The listing builds one solid part. Answer for the finished solid, in the listing's coordinates (mm). A direction names the side the tool comes from. Give positions to 0.01 mm unless a question says otherwise; leave off trailing zeros. Order: outer loops, then holes, each group sorted by start corner. A loop starts at its lowest first (then second) coordinate and runs counter-clockwise, first axis right, second up. Notation, with made-up numbers: (-29.5, 53) - (-7.5, 53) arc R7 ccw to (-7.5, 64) - close; hole circle Ø3 at (82.25, 80.5). An arc over 180 degrees is marked (long way). Use CSV: the item, a comma, the result in double quotes.
```python
from build123d import *

# Parameters (mm, degrees)
CROQUIS1_R                = 4
CROQUIS1_R_2              = 2
SALIENTE_EXTRUIR1_DEPTH   = 4
SALIENTE_EXTRUIR1_2_DEPTH = 4
SALIENTE_EXTRUIR1_3_DEPTH = 4
SALIENTE_EXTRUIR1_4_DEPTH = 4
SALIENTE_EXTRUIR1_5_DEPTH = 4
CROQUIS3_R                = 2
SALIENTE_EXTRUIR4_DEPTH   = 3
CROQUIS4_R                = 4
CROQUIS4_R_2              = 2
CORTAR_EXTRUIR1_DEPTH     = 4
CROQUIS5_R                = 2
SALIENTE_EXTRUIR5_DEPTH   = 3
CROQUIS6_R                = 4
CROQUIS6_R_2              = 2
SALIENTE_EXTRUIR6_DEPTH   = 3


with BuildPart() as part:
    # Croquis1 → Saliente-Extruir1 (new body)
    with BuildSketch(Plane(origin=(0, 0, 0), x_dir=(1, 0, 0), z_dir=(0, 1, 0))):
        with Locations(Location((0, 0, 0), (0, 0, 270))):
            Circle(CROQUIS1_R)
        with Locations(Location((0, 0, 0), (0, 0, 270))):
            Circle(CROQUIS1_R_2, mode=Mode.SUBTRACT)
    extrude(amount=SALIENTE_EXTRUIR1_DEPTH)



with BuildPart() as body_2:
    # Croquis1 → Saliente-Extruir1 2 (new body)
    with BuildSketch(Plane(origin=(0, 0, 0), x_dir=(1, 0, 0), z_dir=(0, 1, 0))):
        with Locations(Location((60.02, 0, 0), (0, 0, 270))):
            Circle(CROQUIS1_R)
        with Locations(Location((60.02, 0, 0), (0, 0, 270))):
            Circle(CROQUIS1_R_2, mode=Mode.SUBTRACT)
    extrude(amount=SALIENTE_EXTRUIR1_2_DEPTH)


with BuildPart() as body_3:
    # Croquis1 → Saliente-Extruir1 3 (new body)
    with BuildSketch(Plane(origin=(0, 0, 0), x_dir=(1, 0, 0), z_dir=(0, 1, 0))):
        with Locations(Location((60.02, -31.02, 0), (0, 0, 270))):
            Circle(CROQUIS1_R)
        with Locations(Location((60.02, -31.02, 0), (0, 0, 270))):
            Circle(CROQUIS1_R_2, mode=Mode.SUBTRACT)
    extrude(amount=SALIENTE_EXTRUIR1_3_DEPTH)


with BuildPart() as body_4:
    # Croquis1 → Saliente-Extruir1 4 (new body)
    with BuildSketch(Plane(origin=(0, 0, 0), x_dir=(1, 0, 0), z_dir=(0, 1, 0))):
        with Locations(Location((0, -31.02, 0), (0, 0, 270))):
            Circle(CROQUIS1_R)
        with Locations(Location((0, -31.02, 0), (0, 0, 270))):
            Circle(CROQUIS1_R_2, mode=Mode.SUBTRACT)
    extrude(amount=SALIENTE_EXTRUIR1_4_DEPTH)


with BuildPart() as body_5:
    # Croquis1 → Saliente-Extruir1 5 (new body)
    with BuildSketch(Plane(origin=(0, 0, 0), x_dir=(1, 0, 0), z_dir=(0, 1, 0))):
        with Locations(Location((30.01, -15.51, 0), (0, 0, 270))):
            Circle(CROQUIS1_R)
        with Locations(Location((30.01, -15.51, 0), (0, 0, 270))):
            Circle(CROQUIS1_R_2, mode=Mode.SUBTRACT)
    extrude(amount=SALIENTE_EXTRUIR1_5_DEPTH)

    # Croquis4 → Cortar-Extruir1 (cut)
    with BuildSketch(Plane.XZ):
        with Locations((30.01, 15.51)):
            Circle(CROQUIS4_R)
        with Locations(Location((30.01, 15.51, 0), (0, 0, 90))):
            Circle(CROQUIS4_R_2, mode=Mode.SUBTRACT)
    extrude(amount=-CORTAR_EXTRUIR1_DEPTH, mode=Mode.SUBTRACT)


with BuildPart() as part_1:
    add(part.part)

    add(body_4.part)  # Saliente-Extruir4 merges body 4

    add(body_2.part)  # Saliente-Extruir4 merges body 2

    add(body_3.part)  # Saliente-Extruir4 merges body 3
    # Croquis3 → Saliente-Extruir4 (add)
    with BuildSketch(Plane(origin=(0, 4, 0), x_dir=(1, 0, 0), z_dir=(0, 1, 0))):
        with BuildLine():
            Line((1.836531919, -34.573470207), (30.01, -20.012640819))
            Line((30.01, -20.012640819), (58.183468081, -34.573470207))
            ThreePointArc((58.183468081, -34.573470207), (63.573470207, -32.856531919), (61.856531919, -27.466529793))
            Line((61.856531919, -27.466529793), (38.722072919, -15.51))
            Line((38.722072919, -15.51), (61.856531919, -3.553470207))
            ThreePointArc((61.856531919, -3.553470207), (63.573470207, 1.836531919), (58.183468081, 3.553470207))
            Line((58.183468081, 3.553470207), (30.01, -11.007359181))
            Line((30.01, -11.007359181), (1.836531919, 3.553470207))
            ThreePointArc((1.836531919, 3.553470207), (-3.553470207, 1.836531919), (-1.836531919, -3.553470207))
            Line((-1.836531919, -3.553470207), (21.297927081, -15.51))
            Line((21.297927081, -15.51), (-1.836531919, -27.466529793))
            ThreePointArc((-1.836531919, -27.466529793), (-3.553470207, -32.856531919), (1.836531919, -34.573470207))
        make_face()
        with Locations(Location((0, -31.02, 0), (0, 0, 270))):
            Circle(CROQUIS3_R, mode=Mode.SUBTRACT)
        with Locations(Location((0, 0, 0), (0, 0, 270))):
            Circle(CROQUIS3_R, mode=Mode.SUBTRACT)
        with BuildLine():
            ThreePointArc((28.01, -15.51), (28.595786438, -14.095786438), (30.01, -13.51))
            ThreePointArc((30.01, -13.51), (31.424213562, -16.924213562), (28.01, -15.51))
        make_face(mode=Mode.SUBTRACT)
        with Locations(Location((60.02, 0, 0), (0, 0, 270))):
            Circle(CROQUIS3_R, mode=Mode.SUBTRACT)
        with Locations(Location((60.02, -31.02, 0), (0, 0, 270))):
            Circle(CROQUIS3_R, mode=Mode.SUBTRACT)
    extrude(amount=SALIENTE_EXTRUIR4_DEPTH)

    # Croquis5 → Saliente-Extruir5 (add)
    with BuildSketch(Plane.XZ.offset(-4)):
        with Locations((30.01, 15.51)):
            Circle(CROQUIS5_R)
    extrude(amount=-SALIENTE_EXTRUIR5_DEPTH)

    # Croquis6 → Saliente-Extruir6 (add)
    # profile 1 of 4: a face of its own
    with BuildSketch(Plane(origin=(0, 7, 0), x_dir=(1, 0, 0), z_dir=(0, 1, 0))):
        with Locations(Location((60.02, 0, 0), (0, 0, 270))):
            Circle(CROQUIS6_R)
        with Locations(Location((60.02, 0, 0), (0, 0, 270))):
            Circle(CROQUIS6_R_2, mode=Mode.SUBTRACT)
    # profile 2 of 4: a face of its own
    with BuildSketch(Plane(origin=(0, 7, 0), x_dir=(1, 0, 0), z_dir=(0, 1, 0))):
        with Locations(Location((0, 0, 0), (0, 0, 270))):
            Circle(CROQUIS6_R)
        with Locations(Location((0, 0, 0), (0, 0, 270))):
            Circle(CROQUIS6_R_2, mode=Mode.SUBTRACT)
    # profile 3 of 4: a face of its own
    with BuildSketch(Plane(origin=(0, 7, 0), x_dir=(1, 0, 0), z_dir=(0, 1, 0))):
        with Locations(Location((0, -31.02, 0), (0, 0, 270))):
            Circle(CROQUIS6_R)
        with Locations(Location((0, -31.02, 0), (0, 0, 270))):
            Circle(CROQUIS6_R_2, mode=Mode.SUBTRACT)
    # profile 4 of 4: a face of its own
    with BuildSketch(Plane(origin=(0, 7, 0), x_dir=(1, 0, 0), z_dir=(0, 1, 0))):
        with Locations(Location((60.02, -31.02, 0), (0, 0, 270))):
            Circle(CROQUIS6_R)
        with Locations(Location((60.02, -31.02, 0), (0, 0, 270))):
            Circle(CROQUIS6_R_2, mode=Mode.SUBTRACT)
    extrude(amount=SALIENTE_EXTRUIR6_DEPTH)


solid = part_1.part
```
Item 1: The part is cut by section C-C (x = 19.5). Give the vertices of the cut face in (y, z).
Taken from the geometry:
outline,"(4, 5.58) - (7, 5.58) - (7, 14.58) - (4, 14.58) - close; (4, 16.44) - (7, 16.44) - (7, 25.44) - (4, 25.44) - close"
Item 2: The part is cut by section D-D (z = 0). Give the vertices of the cut face in (x, y).
Taken from the geometry:
outline,"(-4, 0) - (-2, 0) - (-2, 10) - (-4, 10) - close; (2, 0) - (4, 0) - (4, 4) - (8.71, 4) - (8.71, 7) - (4, 7) - (4, 10) - (2, 10) - close; (51.31, 4) - (56.02, 4) - (56.02, 0) - (58.02, 0) - (58.02, 10) - (56.02, 10) - (56.02, 7) - (51.31, 7) - close; (62.02, 0) - (64.02, 0) - (64.02, 10) - (62.02, 10) - close"
Item 3: The part is cut by section A-A (y = 5.75). Give the vertices of the cut face in (x, z), and give its area (3 significant figures).
Taken from the geometry:
outline,"(-1.84, 3.55) arc R4 ccw to (1.84, -3.55) - (30.01, 11.01) - (58.18, -3.55) arc R4 ccw to (61.86, 3.55) - (38.72, 15.51) - (61.86, 27.47) arc R4 ccw to (58.18, 34.57) - (30.01, 20.01) - (1.84, 34.57) arc R4 ccw to (-1.84, 27.47) - (21.3, 15.51) - close; hole circle Ø4 at (0, 0); hole circle Ø4 at (0, 31.02); hole circle Ø4 at (60.02, 0); hole circle Ø4 at (60.02, 31.02)"
area,"1,050 mm^2"
Item 4: Each of these flat-tipped pins is pushed along its axis until it touches: pin 1 (10 mm diameter, centred on x = 9.5, z = 22.5, fed in from +Y); pin 2 (6 mm diameter, centred on y = 6.5, z = 11, fed in from +X); pin 3 (11.5 mm diameter, centred on x = 20.5, z = 10.5, fed in from -Y); pin 4 (1.5 mm diameter, centred on x = 46, y = 8, fed in from +Z). Where does it stop, or does it pass through?
Taken from the geometry:
pin 1,"y = 7"
pin 2,"x = 53.25"
pin 3,"y = 4"
pin 4,"through"
Item 5: Which of the six approach directions +Z, -Z, +X, -X, +Y, -Y give full straight-line access (tool end or side, diameter ignored) to faces 1 (the face through (50.45, 5.48, 21.57)), 2 (the face through (16.12, 5.48, 3.83)), 3 (the face through (43.9, 5.48, 27.19))?
Taken from the geometry:
face 1,"+X, +Y, -Y"
face 2,"-Z, +Y, -Y"
face 3,"+Z, +Y, -Y"
Item 6: The mould has two halves that part along Z. Classify faces 4 (the face through (44.294, 5.479, 3.625)), 5 (the face through (58.246, 4.93, 0.923)), 6 (the face through (-1, 10, -2)): +Z half, -Z half, draft (parallel to the pull), parting line (faces both ways), or undercut.
Taken from the geometry:
face 4,"-Z half"
face 5,"undercut"
face 6,"draft"
Item 7: Find the intervals of material crossed by line 1 along Z through (x, y) = (60, 8.25); line 2 along Z through (x, y) = (1.5, 5); line 3 along X through (y, z) = (5.5, 29.5), in increasing order.
Taken from the geometry:
line 1,"-4 to -2, 2 to 4, 27.02 to 29.02, 33.02 to 35.02"
line 2,"-3.71 to -1.32, 1.32 to 5.28, 25.74 to 29.7, 32.34 to 34.73"
line 3,"-3.7 to -1.3, 1.3 to 11.65, 48.37 to 58.72, 61.32 to 63.72"
